The listing builds one solid part. Answer for the finished solid, in the listing's coordinates (mm). Face numbers are marked on the shaded views. A direction names the side the tool comes from. Coordinates: 2 decimals unless noted, no trailing zeros. Write each loop counter-clockwise with the first axis right and the second up, starting at its lowest first coordinate (ties: lowest second). Pieces come first, ordered by that corner, then holes.
Autodesk Fusion 360 part; units mm, degrees
sketch "Sketch1" plane through (0, 0, 0) normal (0, 0, 1) x (1, 0, 0)
  circle A0 centre (0, 0) radius 15
  dimension "d2" = 30
extrude "Extrude1" add sketch "Sketch1" along normal blind 50
sketch "Sketch2" plane through (0, 0, 50) normal (0, 0, 1) x (-1, 0, 0)
  circle A0 centre (0, 0) radius 15
  circle A1 centre (0, 0) radius 12.5
  dimension "d5" = 25
extrude "Extrude2" cut sketch "Sketch2" against normal blind 45 contours A1
sketch "Sketch4" plane through (0, 0, 50) normal (0, 0, 1) x (-1, 0, 0)
  circle A0 centre (0, 0) radius 12.5
  circle A1 centre (0, 0) radius 15
  circle A2 centre (0, 0) radius 15
  circle A3 centre (0, 0) radius 5.5
  dimension "d8" = 11
extrude "Extrude3" add sketch "Sketch4" against normal blind 5 contours A0
sketch "Sketch5" plane through (0, 0, 50) normal (0, 0, 1) x (-1, 0, 0)
  circle A0 centre (0, 0) radius 5.5
  circle A1 centre (0, 0) radius 15
  circle A2 centre (0, 0) radius 12.5
  circle A3 centre (0, 0) radius 7.5
  line L0 (0, 0) -> (12.5, 0) construction
  line L1 (0, 0) -> (-10.8253, 6.25)
  line L2 (0, 0) -> (12.5, 0) construction
  line L3 (0, 0) -> (-10.8253, -6.25)
  line L4 (0, 0) -> (12.5, 0) construction
  line L5 (0, 0) -> (10.8253, 6.25)
  line L6 (-10.8253, 6.25) -> (14.1746, 6.25) construction
  line L7 (0, 0) -> (10.8253, -6.25)
  line L8 (0, 0) -> (12.5, 0) construction
  dimension "d11" = 25
  dimension "d12" = 15
  dimension "d14" = 150
  dimension "d15" = 150
  dimension "d18" = 30
extrude "Extrude4" cut sketch "Sketch5" against normal blind 5 contours A2 A3 L5 L7 | A2 A3 L1 L3
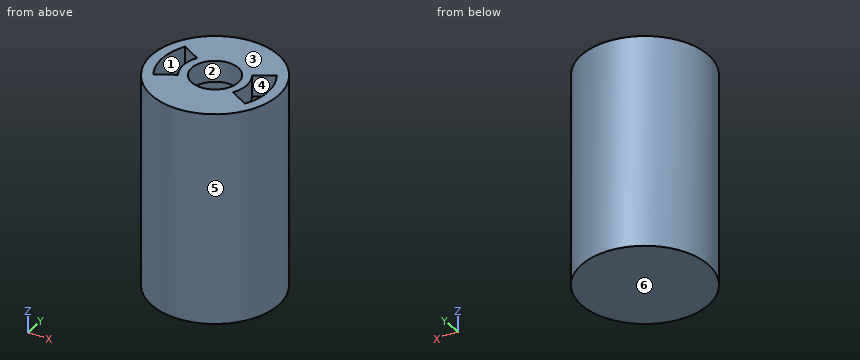
Q1. Find the intervals of material crossed by probe 1 along Y at (x, z) = (0.5, 15.5); probe 2 along Y at (x, z) = (0, 48.8); probe 3 along Z at (x, y) = (-0.25, -0.5), in increasing order.
Answers below:
probe 1: y = -14.99 to -12.49, 12.49 to 14.99
probe 2: y = -15 to -5.5, 5.5 to 15
probe 3: z = 0 to 5
Q2. Given pin 1 (4 mm diameter, centred on x = 10, z = 14.5, fed in from +Y); pin 2 (1.5 mm diameter, centred on x = -3, z = 26, fed in from -Y); pin 3 (12 mm diameter, centred on y = -10, z = 24, fed in from -X), each flat-ended and moving along its own axis, determine where each tip first touches the part or whether it passes through.
Answers below:
pin 1: stops at y = 12.69
pin 2: stops at y = -14.83
pin 3: stops at x = -14.46
Q3. Determine the mould class of the marked faces 4, 5 and 6 for opening direction Y: released by +Y, released by -Y, zero draft, split by the parting line, or undercut.
Answers below:
face 4: undercut
face 5: split by the parting line
face 6: zero draft
Q4. Which of the six approach directions +Z, -Z, +X, -X, +Y, -Y give full straight-line access (tool end or side, diameter ignored) to the marked faces 1, 2 and 3?
Answers below:
face 1: none
face 2: +Z
face 3: +Z, +X, -X, +Y, -Y
Q5. The part is cut by section B-B, the plane x = 0. Write down the section's boundary in (y, z), then the cut area to 3 significant figures.
Answers below:
outline: (-15, 0) - (15, 0) - (15, 50) - (5.5, 50) - (5.5, 45) - (12.5, 45) - (12.5, 5) - (-12.5, 5) - (-12.5, 45) - (-5.5, 45) - (-5.5, 50) - (-15, 50) - close
area: 445 mm2
Q6. The part is cut by section D-D, the plane y = -11.75. Write down the section's boundary in (x, z).
Answers below:
outline: (-9.32, 0) - (9.32, 0) - (9.32, 50) - (-9.32, 50) - close; hole (-4.26, 5) - (4.26, 5) - (4.26, 45) - (-4.26, 45) - close
Q7. The part is cut by section A-A, the plane y = 0. Write down the section's boundary in (x, z).
Answers below:
outline: (-15, 0) - (15, 0) - (15, 50) - (12.5, 50) - (12.5, 5) - (-12.5, 5) - (-12.5, 50) - (-15, 50) - close; (-7.5, 45) - (-5.5, 45) - (-5.5, 50) - (-7.5, 50) - close; (5.5, 45) - (7.5, 45) - (7.5, 50) - (5.5, 50) - close
Q8. The part is cut by section C-C, the plane z = 16. Write down the section's boundary in (x, y).
Answers below:
outline: circle Ø30 at (0, 0); hole circle Ø25 at (0, 0)
